from build123d import *

# Parameters (mm, degrees)
F0_W     = 140
F0_H     = 60
F1_DEPTH = 25
F2_R     = 10
F5_DEPTH = 10
F4_R     = 10
F6_DEPTH = 41.8
F3_R     = 10
F7_DEPTH = 10


with BuildPart() as f1:
    # F0 (on Top) → F1 (new body)
    with BuildSketch(Plane.XY):
        Rectangle(F0_W, F0_H)
    extrude(amount=F1_DEPTH)

    # F2 (on face) → F5 (join)
    with BuildSketch(Plane.XY.offset(25)):
        with Locations((-48.220878, 0)):
            Circle(F2_R)
    extrude(amount=F5_DEPTH)

    # F4 (on face) → F6 (cut)
    with BuildSketch(Plane.XY.offset(25)):
        Circle(F4_R)
    extrude(amount=-F6_DEPTH, mode=Mode.SUBTRACT)

    # F3 (on face) → F7 (cut)
    with BuildSketch(Plane.XY.offset(25)):
        with Locations((40, 0)):
            Circle(F3_R)
    extrude(amount=-F7_DEPTH, mode=Mode.SUBTRACT)


solid = f1.part
The model under review builds one solid part; all positions refer to its coordinate system, in mm. A direction names the side the tool comes from. Give positions to 0.01 mm unless a question says otherwise; leave off trailing zeros. Order: outer loops, then holes, each group sorted by start corner. A loop starts at its lowest first (then second) coordinate and runs counter-clockwise, first axis right, second up. Notation, with made-up numbers: M 15.25,-27 L 23.25,-27 A14 ccw 23.25,-15 Z; hole C 38.5,58.25 d8. An arc over 180 degrees is marked long. Answer in a Markdown table with one row per item. Add a question column.
1. Add section A-A on y = 0. State the section outline as (x, z) points, plus the area to 3 significant figures.
2. Add section C-C on x = 40. State the section outline as (y, z) points.
3. Add section B-B on z = 12. State the section outline as (x, y) points, plus the area to 3 significant figures.
4. Add section D-D on z = 20. State the section outline as (x, y) points.
5. Mouldability with a two-part tool opening along Y and no side actions: class faces 3 (the cylindrical face through (-2.17, -9.76, 12.68)), 4 (the flat face through (-70, 0, 12)), 5 (the flat face through (40, 0, 15)), 6 (the flat face through (-1, 30, 12)) as released by +Y, released by -Y, zero draft, split by the parting line, or undercut.
6. For pin 1 Ø4 at (x, y) = (17, -1.5) entering from +Z; pin 2 Ø6 at (x, y) = (38.5, 1) entering from +Z; pin 3 Ø2 at (x, y) = (-42, 9) entering from -Z, all flat-tipped, find the tip position at first contact; note any pin that passes through.
7. Machinability: for faces 1 (the flat face through (-1, 14, 0)), 2 (the cylindrical face through (30, 0, 20)), which of the approach directions +Z, -Z, +X, -X, +Y, -Y give a long, thin tool a straight path to every point of the face, cutting with its end or side? Answer none if there is none.
8. To check wall thickness, follow line 1 along Y through (x, z) = (0, 13); line 2 along X through (y, z) = (-4.5, 23); line 3 along Z through (x, y) = (-48, 15). State the ranges of each line that lie inside material, in increasing order.
The answers:
| question | item | result |
|---|---|---|
| 1 | outline | M -70,0 L -10,0 L -10,25 L -38.22,25 L -38.22,35 L -58.22,35 L -58.22,25 L -70,25 Z; M 10,0 L 70,0 L 70,25 L 50,25 L 50,15 L 30,15 L 30,25 L 10,25 Z |
| 1 | area | 3,000 mm2 |
| 2 | outline | M -30,0 L 30,0 L 30,25 L 10,25 L 10,15 L -10,15 L -10,25 L -30,25 Z |
| 3 | outline | M -70,-30 L 70,-30 L 70,30 L -70,30 Z; hole C 0,0 d20 |
| 3 | area | 8,090 mm2 |
| 4 | outline | M -70,-30 L 70,-30 L 70,30 L -70,30 Z; hole C 0,0 d20; hole C 40,0 d20 |
| 5 | face 3 | undercut |
| 5 | face 4 | zero draft |
| 5 | face 5 | undercut |
| 5 | face 6 | released by +Y |
| 6 | pin 1 | z = 25 |
| 6 | pin 2 | z = 15 |
| 6 | pin 3 | z = 0 |
| 7 | face 1 | -Z, +X, -X, +Y, -Y |
| 7 | face 2 | +Z |
| 8 | line 1 | -30 to -10, 10 to 30 |
| 8 | line 2 | -70 to -8.93, 8.93 to 31.07, 48.93 to 70 |
| 8 | line 3 | 0 to 25 |
